```python
from build123d import *

# Parameters (mm, degrees)
EXTRUDE_START       = 4
SKETCH_2_R          = 8.114467409
EXTRUDE_1_DEPTH     = 4
SKETCH_4_R          = 9.25
CUT_EXTRUDE_1_DEPTH = 5
SKETCH_5_OUTSIDE_W  = 43.9
SKETCH_5_OUTSIDE_H  = 52.854
CUT_EXTRUDE_7_DEPTH = 4
EXTRUDE_3_DEPTH     = 5
SKETCH_9_W          = 20
SKETCH_9_H          = 4
EXTRUDE_4_DEPTH     = 21
SKETCH_11_W         = 20
SKETCH_11_H         = 4
EXTRUDE_5_DEPTH     = 4
FILLET_1_R          = 5


with BuildPart() as part:
    # Sketch 1 → Revolve 1 (revolve)
    with BuildSketch(Plane.XY, mode=Mode.PRIVATE) as revolve_1_sk:
        Polygon((0, 0), (11, 0), (15, 5.5), (15, 6), (10, 6), (10, 7.5), (15, 7.5), (15, 11.5), (10, 11.5), (10, 24.5), (6.326264721, 24.5), (6.326264721, 28.5), (8, 28.5), (8, 33.5), (0, 33.5), align=None)
    revolve(revolve_1_sk.sketch.rotate(Axis((0, 38.134324324, 0), (0, -1, 0)), 90), axis=Axis((0, 38.134324324, 0), (0, -1, 0)))

    # Sketch 2 → Extrude 1 (add)
    with BuildSketch(Plane(origin=(0, 24.5, 0), x_dir=(1, 0, 0), z_dir=(0, 1, 0)).offset(EXTRUDE_START)):
        with BuildLine():
            Line((-8, 6), (-10, 19.953992765))
            Line((-10, 19.953992765), (-10, 23.953992765))
            Line((-10, 23.953992765), (10, 23.953992765))
            Line((10, 23.953992765), (10, 19.953992765))
            Line((10, 19.953992765), (8, 6))
            ThreePointArc((8, 6), (0, -10), (-8, 6))
        make_face()
        with Locations(Location((0, 0, 0), (0, 0, 270))):
            Circle(SKETCH_2_R, mode=Mode.SUBTRACT)
    extrude(amount=-EXTRUDE_1_DEPTH)

    # Sketch 4 → Cut-Extrude 1 (cut)
    with BuildSketch(Plane.XZ):
        with Locations(Location((0, 0, 0), (0, 0, 270))):
            Circle(SKETCH_4_R)
    extrude(amount=-CUT_EXTRUDE_1_DEPTH, mode=Mode.SUBTRACT)

    # Sketch 5 outside → Cut-Extrude 7 (cut)
    with BuildSketch(Plane(origin=(0, 11.5, 0), x_dir=(1, 0, 0), z_dir=(0, 1, 0))):
        with Locations((0, 4.477)):
            Rectangle(SKETCH_5_OUTSIDE_W, SKETCH_5_OUTSIDE_H)
        Polygon((0, -15), (12.990381057, -7.5), (12.990381057, 7.5), (0, 15), (-12.990381057, 7.5), (-12.990381057, -7.5), align=None, mode=Mode.SUBTRACT)
    extrude(amount=-CUT_EXTRUDE_7_DEPTH, mode=Mode.SUBTRACT)

    # Sketch 6 → Extrude 3 (add)
    with BuildSketch(Plane.XZ.offset(-5)):
        Polygon((-4.5, -3.897114317), (0, 3.897114317), (4.5, -3.897114317), align=None)
    extrude(amount=EXTRUDE_3_DEPTH)



with BuildPart() as body_2:
    # Sketch 9 → Extrude 4 (new body)
    with BuildSketch(Plane(origin=(0, 0, -23.953992765), x_dir=(-1, 0, 0), z_dir=(0, 0, -1))):
        with Locations((0, 30.5)):
            Rectangle(SKETCH_9_W, SKETCH_9_H)
    extrude(amount=EXTRUDE_4_DEPTH)


with BuildPart() as part_1:
    add(part.part)

    add(body_2.part)  # Extrude 5 merges body 2
    # Sketch 11 → Extrude 5 (add)
    with BuildSketch(Plane.XY.offset(-23.953992765)):
        with Locations((0, 30.5)):
            Rectangle(SKETCH_11_W, SKETCH_11_H)
    extrude(amount=EXTRUDE_5_DEPTH)

    # Fillet 1
    fillet_1_edges = [part_1.edges().sort_by_distance(p)[0] for p in [
        (10, 30.5, -44.953992765),
        (-10, 30.5, -44.953992765),
    ]]
    fillet(fillet_1_edges, radius=FILLET_1_R)


solid = part_1.part
```
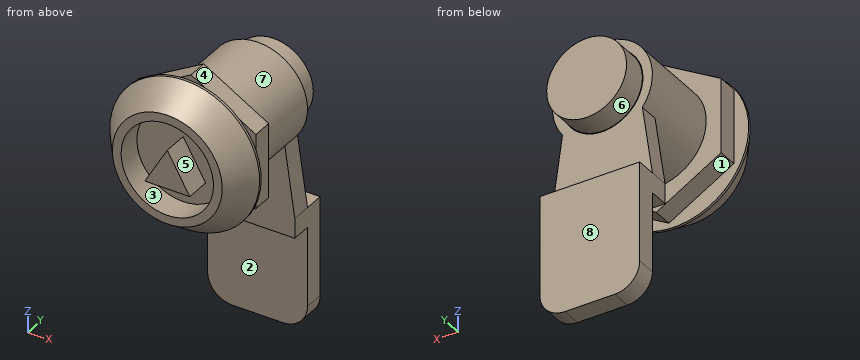
CAD build for the part. Positions are in the model's coordinates, mm. Face numbers are marked on the shaded views. A direction names the side the tool comes from. Give positions to 0.01 mm unless a question says otherwise; leave off trailing zeros. Order: outer loops, then holes, each group sorted by start corner. A loop starts at its lowest first (then second) coordinate and runs counter-clockwise, first axis right, second up. Notation, with made-up numbers: M 29,49 L 37,49 A11 cw 37,59 Z; hole C 79.25,27.5 d1. An arc over 180 degrees is marked long. Put each result on its own line as item: value. Start each with the question number.
(1) Which spindle directions (+Z, -Z, +X, -X, +Y, -Y) get a long thin tool onto all of the face, cutting with end or side? Do the marked faces 4, 5, 6, 7 and 8. Say none if no direction does.
(2) Drill centre lines: line 1 along X through (y, z) = (1.15, 0); line 2 along X through (y, z) = (3.9, 0); line 3 along X through (y, z) = (23, 8). Where is each one in solid material? Low to high.
(3) Mould opens along Z. For the marked faces 1, 2 and 3 say: +Z half, -Z half, draft (parallel to the pull), parting line (faces both ways), or undercut.
(4) Flat gauge pins, fed straight in: pin 1 Ø16 at (x, z) = (-3.5, -34.5) entering from +Y; pin 2 Ø4.5 at (y, z) = (9.5, 3.5) entering from -X; pin 3 Ø3 at (x, y) = (2.5, 30.5) entering from +Z. Where does each tip first touch, or does it go through?
(5) Saw through at B-B, the plane y = 9. Write the cut outline in (x, z).
(6) Saw through at C-C, the plane y = 15.5. Write the cut outline in (x, z).
(7) Saw through at A-A, the plane y = 26.5. Write the cut outline in (x, z).
Check result:
1. face 4: +Z, +X, +Y
1. face 5: -Y
1. face 6: +Y
1. face 7: none
1. face 8: -Z, +X, -X, +Y
2. line 1: x = -11.84 to -9.25, -2.25 to 2.25, 9.25 to 11.84
2. line 2: x = -13.84 to -9.25, -2.25 to 2.25, 9.25 to 13.84
2. line 3: x = -6 to 6
3. face 1: -Z half
3. face 2: draft
3. face 3: undercut
4. pin 1: stops at y = 32.5
4. pin 2: stops at x = -12.99
4. pin 3: stops at z = 7.94
5. outline: M -12.99,-7.5 L 0,-15 L 12.99,-7.5 L 12.99,7.5 L 0,15 L -12.99,7.5 Z
6. outline: C 0,0 d20
7. outline: M -10,-23.95 L 10,-23.95 L 10,-19.95 L 8,-6 A10 ccw long -8,-6 L -10,-19.95 Z; C 0,0 d12.65; hole C 0,0 d16.23
